Model file for the job. Use its own axes, mm. A direction names the side the tool comes from. Give positions to 0.01 mm unless a question says otherwise; leave off trailing zeros. Write each loop counter-clockwise with the first axis right and the second up, starting at its lowest first coordinate (ties: lowest second). Pieces come first, ordered by that corner, then holes.
```python
from build123d import *

# Parameters (mm, degrees)
SKETCH2_W           = 215
SKETCH2_H           = 78.5
SKETCH2_W_2         = 205
SKETCH2_H_2         = 68.5
BOSS_EXTRUDE1_DEPTH = 50
SKETCH2_2_W         = 205
SKETCH2_2_H         = 68.5
BOSS_EXTRUDE2_DEPTH = 2.5
FILLET1_SIZE        = 7


with BuildPart() as part:
    # Sketch2 → Boss-Extrude1 (new, symmetric)
    with BuildSketch(Plane(origin=(0, 0, 0), x_dir=(1, 0, 0), z_dir=(0, 1, 0))):
        Rectangle(SKETCH2_W, SKETCH2_H)
        Rectangle(SKETCH2_W_2, SKETCH2_H_2, mode=Mode.SUBTRACT)
    extrude(amount=BOSS_EXTRUDE1_DEPTH, both=True)

    # Sketch2<2> → Boss-Extrude2 (add, symmetric)
    with BuildSketch(Plane(origin=(0, 0, 0), x_dir=(1, 0, 0), z_dir=(0, 1, 0))):
        Rectangle(SKETCH2_2_W, SKETCH2_2_H)
    extrude(amount=BOSS_EXTRUDE2_DEPTH, both=True)

    # Fillet1
    # a fillet whose section is not a circle: 7 mm, written as the material it takes off along each edge
    with BuildSketch(Plane(origin=(-107.5, -67.5, -39.25), x_dir=(1, 0, 0), z_dir=(0, 1, 0)), Plane(origin=(-107.5, -67.5, 39.25), x_dir=(0, 0, -1), z_dir=(0, 1, 0)), Plane(origin=(107.5, 67.5, 39.25), x_dir=(0, 0, -1), z_dir=(0, -1, 0)), Plane(origin=(107.5, 67.5, -39.25), x_dir=(-1, 0, 0), z_dir=(0, -1, 0))) as fillet1_piece_1:
        with BuildLine():
            add(Edge.make_bspline([(FILLET1_SIZE, 0), (FILLET1_SIZE * 0.831801948466, 0), (FILLET1_SIZE * 0.663603896932, 0), (FILLET1_SIZE * 0.292893218813, -FILLET1_SIZE * 0.0716919198361), (FILLET1_SIZE * 0.0716919198361, -FILLET1_SIZE * 0.292893218813), (0, -FILLET1_SIZE * 0.663603896932), (0, -FILLET1_SIZE * 0.831801948466), (0, -FILLET1_SIZE)], knots=[0, 0, 0, 0, 0, 0, 0.5, 0.5, 1, 1, 1, 1, 1, 1], degree=5))
            Line((0, -FILLET1_SIZE), (0, 0))
            Line((0, 0), (FILLET1_SIZE, 0))
        make_face()
    extrude(amount=135, mode=Mode.SUBTRACT)


solid = part.part
```
1. Slice it at A-A, the plane z = -1. Write the cut outline in (x, y).
Calculated:
outline: (-107.5, -50) - (-102.5, -50) - (-102.5, -2.5) - (102.5, -2.5) - (102.5, -50) - (107.5, -50) - (107.5, 50) - (102.5, 50) - (102.5, 2.5) - (-102.5, 2.5) - (-102.5, 50) - (-107.5, 50) - close
2. Pull direction Z, two halves, no side cores. Call faces 4 (the flat face through (-8, -50, 35)), 5 (the flat face through (-102.5, -26, 0)), 6 (the flat face through (-1, 1, -39.25)): +Z half, -Z half, draft (parallel to the pull), parting line (faces both ways), or undercut.
Calculated:
face 4: draft
face 5: undercut
face 6: -Z half
3. Probe probe 1 along Z at (x, y) = (12, 7.5); probe 2 along X at (y, z) = (-3.5, 28.5); probe 3 along Y at (x, z) = (-84.5, 30). List the from-to ranges inside material, lowest first.
Calculated:
probe 1: z = -39.25 to -34.25, 34.25 to 39.25
probe 2: x = -107.5 to -102.5, 102.5 to 107.5
probe 3: y = -2.5 to 2.5
4. Slice it at B-B, the plane x = 38.5. Write the cut outline in (y, z).
Calculated:
outline: (-50, -39.25) - (50, -39.25) - (50, -34.25) - (2.5, -34.25) - (2.5, 34.25) - (50, 34.25) - (50, 39.25) - (-50, 39.25) - (-50, 34.25) - (-2.5, 34.25) - (-2.5, -34.25) - (-50, -34.25) - close
5. Pin check, flat tips, straight feed: P1, Ø10, axis at x = 2, z = -21, coming from the +Y side; P2, Ø1, axis at x = -79, z = 24.5, coming from the -Y side. Stop position of each tip, or through.
Calculated:
P1: stops at y = 2.5
P2: stops at y = -2.5
6. Which spindle directions (+Z, -Z, +X, -X, +Y, -Y) get a long thin tool onto all of the face, cutting with end or side? Do faces 1 (the flat face through (102.5, 27, 0)), 2 (the flat face through (-8, 50, 35)), 3 (the flat face through (-1, -2.5, 0)). Say none if no direction does.
Calculated:
face 1: +Y
face 2: +Z, -Z, +X, -X, +Y
face 3: -Y
